Can you work these out from the model? Positions are in its coordinate system, mm. Face numbers are marked on the shaded views. A direction names the side the tool comes from. Coordinates: 2 decimals unless noted, no trailing zeros. Loops run counter-clockwise (first coordinate to the right, second up) from the corner with the lowest first, then second, coordinate; pieces in that order, holes last. Notation, with made-up numbers: (-32, 54.5) -> (26, 54.5) arc R17 cw to (26, 81.5) -> close; hole circle Ø7 at (9.25, 75.25). An arc over 180 degrees is marked (long way). Put each result on its own line as item: value. Start each with the question number.
Item 1: Will these pins go through, and if not, where does the flat tip stop? P1, Ø1, axis at x = -22.5, z = 7.5, coming from the +Y side; P2, Ø1.5, axis at x = -27.5, y = 17, coming from the -Z side.
Item 2: If we section it at B-B on z = 10: Please give me the cut outline in (x, y).
Item 3: Please list where these lines run through material, in increasing order: L1, parallel to X at y = 34, z = 15.5; L2, parallel to Z at x = -21, y = 26.5. Write a range as from..to.
Item 4: If we section it at A-A on y = 20: Please give me the cut outline in (x, z), plus the area to 3 significant figures.
Item 5: If we section it at D-D on z = 25.5: Please give me the cut outline in (x, y).
Item 6: If we section it at C-C on y = 8.5: Please give me the cut outline in (x, z), plus the area to 3 significant figures.
Item 7: We'd pull the mould along X, two halves only. Please class the marked faces 3, 4 and 5: pulls with the +X half, pulls with the -X half, needs draft (parallel to the pull), parting line crosses it, or undercut.
Item 8: For the marked faces 1 and 2, which set-ups out of +Z, -Z, +X, -X, +Y, -Y let a thin tool reach every point of the face, with its end or its side?
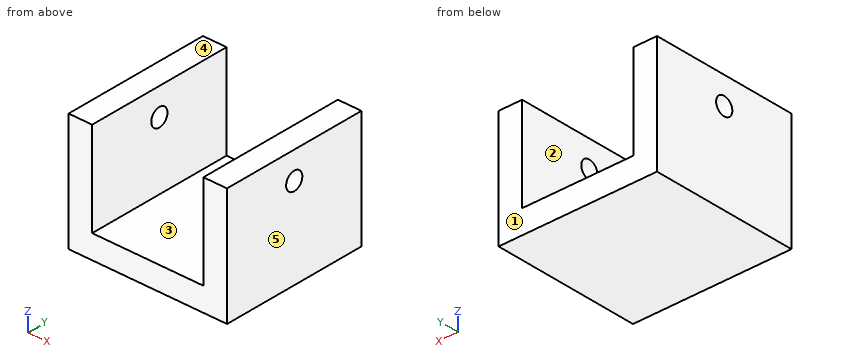
Autodesk Inventor part; units mm, degrees
ref_plane "YZ Plane" through (0, 0, 0) normal (1, 0, 0) x (0, 1, 0)
ref_plane "XZ Plane" through (0, 0, 0) normal (0, 1, 0) x (-1, 0, 0)
ref_plane "XY Plane" through (0, 0, 0) normal (0, 0, 1) x (1, 0, 0)
sketch "Sketch1" plane through (0, 0, 0) normal (0, 0, 1) x (1, 0, 0)
  line L0 (0, 0) -> (-42.672, 0)
  line L1 (-42.672, 0) -> (-42.672, 40)
  line L2 (-42.672, 40) -> (0, 40)
  line L3 (0, 40) -> (0, 0)
  dimension "d0" = 42.672
  dimension "d1" = 40
extrude "Extrusion1" add sketch "Sketch1" along normal blind 6.35
sketch "Sketch2" plane through (0, 0, 6.35) normal (0, 0, 1) x (1, 0, 0)
  line L0 (-42.672, 0) -> (0, 0)
  line L1 (-42.672, 40) -> (-36.322, 40)
  line L2 (-36.322, 40) -> (-36.322, 0)
  line L3 (-36.322, 0) -> (-42.672, 0)
  line L4 (-42.672, 0) -> (-42.672, 40)
  dimension "d4" = 6.35
extrude "Extrusion2" add sketch "Sketch2" along normal blind 25.4
sketch "Sketch3" plane through (0, 0, 6.35) normal (0, 0, 1) x (1, 0, 0)
  line L0 (-36.322, 0) -> (0, 0)
  line L1 (0, 40) -> (-6.35, 40)
  line L2 (-6.35, 40) -> (-6.35, 0)
  line L3 (-6.35, 0) -> (0, 0)
  line L4 (0, 0) -> (0, 40)
  dimension "d7" = 6.35
extrude "Extrusion3" add sketch "Sketch3" along normal blind 25.4
sketch "Sketch4" plane through (0, 0, 0) normal (1, 0, 0) x (0, 0, -1)
  circle A0 centre (-24.4119, 20) radius 2.413
  dimension "d10" = 4.826
extrude "Extrusion4" cut sketch "Sketch4" against normal blind 76.2
properties part number "LiftBase2" material "Aluminum 6061"
Solutions:
1. P1: through
1. P2: z = 0
2. outline: (-42.67, 0) -> (-36.32, 0) -> (-36.32, 40) -> (-42.67, 40) -> close; (-6.35, 0) -> (0, 0) -> (0, 40) -> (-6.35, 40) -> close
3. L1: -42.67..-36.32, -6.35..0
3. L2: 0..6.35
4. outline: (-42.67, 0) -> (0, 0) -> (0, 22) -> (-6.35, 22) -> (-6.35, 6.35) -> (-36.32, 6.35) -> (-36.32, 22) -> (-42.67, 22) -> close; (-42.67, 26.82) -> (-36.32, 26.82) -> (-36.32, 31.75) -> (-42.67, 31.75) -> close; (-6.35, 26.82) -> (0, 26.82) -> (0, 31.75) -> (-6.35, 31.75) -> close
4. area: 532 mm^2
5. outline: (-42.67, 0) -> (-36.32, 0) -> (-36.32, 17.85) -> (-42.67, 17.85) -> close; (-42.67, 22.15) -> (-36.32, 22.15) -> (-36.32, 40) -> (-42.67, 40) -> close; (-6.35, 0) -> (0, 0) -> (0, 17.85) -> (-6.35, 17.85) -> close; (-6.35, 22.15) -> (0, 22.15) -> (0, 40) -> (-6.35, 40) -> close
6. outline: (-42.67, 0) -> (0, 0) -> (0, 31.75) -> (-6.35, 31.75) -> (-6.35, 6.35) -> (-36.32, 6.35) -> (-36.32, 31.75) -> (-42.67, 31.75) -> close
6. area: 594 mm^2
7. face 3: undercut
7. face 4: needs draft
7. face 5: pulls with the +X half
8. face 1: +Z, -Z, +X, -X, +Y
8. face 2: +Z, +Y, -Y
